Model file for the job. Use its own axes, mm. A direction names the side the tool comes from. Round coordinates to 2 decimals unless told otherwise and drop trailing zeros. Order: outer loops, then holes, each group sorted by start corner. A loop starts at its lowest first (then second) coordinate and runs counter-clockwise, first axis right, second up. Notation, with made-up numbers: (45.25, 65) - (60.25, 65) arc R29 cw to (60.25, 94) - close; hole circle Ø8 at (-26, 0). An arc over 180 degrees is marked (long way). Put each result on its own line as item: value. Start each with the question number.
Item 1: Which spindle directions (+Z, -Z, +X, -X, +Y, -Y) get a long thin tool onto all of the face, cutting with end or side? Do faces 4 (the face through (-73, -25.5, 3)), 5 (the face through (-45, -12, 3)), 6 (the face through (45, -68, 3)), 7 (the face through (-70, 12, 3)), 8 (the face through (15, -68, 3)). Say none if no direction does.
Item 2: Saw through at C-C on y = -33.5. List the corners of the cut face in (x, z).
Item 3: Pin check, flat tips, straight feed: pin 1 Ø2.5 at (y, z) = (12, 3) entering from +X; pin 2 Ø1.5 at (x, z) = (-47, 4) entering from -Y; pin 3 Ø1.5 at (x, z) = (-73.5, 2.5) entering from -Y. Stop position of each tip, or through.
Item 4: Saw through at D-D on x = -49.5. List the corners of the cut face in (y, z), plus the area to 3 significant figures.
Item 5: Saw through at A-A on y = -14. List the corners of the cut face in (x, z), plus the area to 3 significant figures.
Item 6: Mould opens along X. For faces 1 (the face through (72, 4.5, 3)), 2 (the face through (45, -13, 3)), 3 (the face through (-75, -10, 2)) say: pulls with the +X half, pulls with the -X half, needs draft (parallel to the pull), parting line crosses it, or undercut.
Item 7: Saw through at B-B on z = 4.15. List the corners of the cut face in (x, y), plus the area to 4 significant figures.
Item 8: Probe probe 1 along X at (y, z) = (-15, 0.6); probe 2 along X at (y, z) = (11, 3.05); probe 3 along Y at (x, z) = (41, 1). List the from-to ranges inside material, lowest first.
Autodesk Inventor part; units mm, degrees
ref_plane "YZ Plane" through (0, 0, 0) normal (1, 0, 0) x (0, 1, 0)
ref_plane "XZ Plane" through (0, 0, 0) normal (0, 1, 0) x (-1, 0, 0)
ref_plane "XY Plane" through (0, 0, 0) normal (0, 0, 1) x (1, 0, 0)
sketch "Sketch1" plane through (0, 0, 0) normal (0, 0, 1) x (1, 0, 0)
  line L0 (0, 2.8582) -> (0, -2.8582) construction
  line L1 (-5.7775, 0) -> (5.7775, 0) construction
  line L2 (-75, -70.5) -> (75, -70.5)
  line L3 (75, -70.5) -> (75, 70.5)
  line L4 (75, 70.5) -> (-75, 70.5)
  line L5 (-75, 70.5) -> (-75, -70.5)
  line L6 (-75, -70.5) -> (75, 70.5) construction
  line L7 (75, -70.5) -> (-75, 70.5) construction
  point P0 (0, 0)
  point P1 (0, 0)
  dimension "d0" = 150
  dimension "d1" = 141
extrude "Extrusion1" add sketch "Sketch1" along normal blind 5
sketch "Sketch2" plane through (0, 0, 5) normal (0, 0, 1) x (1, 0, 0)
  line L0 (-75, -70.5) -> (75, -70.5)
  line L1 (0, -70.5) -> (-15, -70.5)
  line L2 (-15, -70.5) -> (15, -70.5)
  line L3 (15, -70.5) -> (45, -70.5)
  line L4 (-15, -70.5) -> (-45, -70.5)
  line L5 (-15, -70.5) -> (15, -70.5)
  line L6 (15, -70.5) -> (15, -65.5)
  line L7 (15, -65.5) -> (-15, -65.5)
  line L8 (-15, -65.5) -> (-15, -70.5)
  line L9 (75, -70.5) -> (75, 70.5)
  line L10 (45, -70.5) -> (75, -70.5)
  line L11 (75, -70.5) -> (75, -65.5)
  line L12 (75, -65.5) -> (45, -65.5)
  line L13 (45, -65.5) -> (45, -70.5)
  line L14 (-75, 70.5) -> (-75, -70.5)
  line L15 (-45, -70.5) -> (-75, -70.5)
  line L16 (-75, -70.5) -> (-75, -65.5)
  line L17 (-75, -65.5) -> (-45, -65.5)
  line L18 (-45, -65.5) -> (-45, -70.5)
  line L19 (75, -70.5) -> (75, -55.5)
  line L20 (75, -55.5) -> (75, -25.5)
  line L21 (75, -25.5) -> (75, 4.5)
  line L22 (75, 4.5) -> (75, 34.5)
  line L23 (75, 34.5) -> (75, 64.5)
  line L24 (75, -25.5) -> (70, -25.5)
  line L25 (70, -25.5) -> (70, 4.5)
  line L26 (70, 4.5) -> (75, 4.5)
  line L27 (75, 4.5) -> (75, -25.5)
  line L28 (75, 70.5) -> (-75, 70.5)
  line L29 (75, 34.5) -> (70, 34.5)
  line L30 (70, 34.5) -> (70, 70.5)
  line L31 (70, 70.5) -> (75, 70.5)
  line L32 (75, 70.5) -> (75, 34.5)
  line L33 (-75, -25.5) -> (-70, -25.5)
  line L34 (-70, -25.5) -> (-70, 4.5)
  line L35 (-70, 4.5) -> (-75, 4.5)
  line L36 (-75, 4.5) -> (-75, -25.5)
  line L37 (-75, 34.5) -> (-70, 34.5)
  line L38 (-70, 34.5) -> (-70, 70.5)
  line L39 (-70, 70.5) -> (-75, 70.5)
  line L40 (-75, 70.5) -> (-75, 34.5)
  line L41 (0, 70.5) -> (-15, 70.5)
  line L42 (-15, 70.5) -> (15, 70.5)
  line L43 (15, 70.5) -> (45, 70.5)
  line L44 (-15, 70.5) -> (-45, 70.5)
  line L45 (-75, 70.5) -> (-45, 70.5)
  line L46 (-45, 70.5) -> (-45, 65.5)
  line L47 (-45, 65.5) -> (-75, 65.5)
  line L48 (-75, 65.5) -> (-75, 70.5)
  line L49 (-15, 70.5) -> (15, 70.5)
  line L50 (15, 70.5) -> (15, 65.5)
  line L51 (15, 65.5) -> (-15, 65.5)
  line L52 (-15, 65.5) -> (-15, 70.5)
  line L53 (45, 70.5) -> (75, 70.5)
  line L54 (75, 70.5) -> (75, 65.5)
  line L55 (75, 65.5) -> (45, 65.5)
  line L56 (45, 65.5) -> (45, 70.5)
  line L57 (-75, -25.5) -> (-70, -25.5)
  line L58 (-70, -25.5) -> (-70, -70.5)
  line L59 (-70, -70.5) -> (-75, -70.5)
  line L60 (-75, -70.5) -> (-75, -25.5)
  line L61 (-75, 4.5) -> (-70, 4.5)
  line L62 (-70, 4.5) -> (-70, 34.5)
  line L63 (-70, 34.5) -> (-75, 34.5)
  line L64 (-75, 34.5) -> (-75, 4.5)
  line L65 (70, 34.5) -> (75, 34.5)
  line L66 (75, 34.5) -> (75, 4.5)
  line L67 (75, 4.5) -> (70, 4.5)
  line L68 (70, 4.5) -> (70, 34.5)
  line L69 (70, -25.5) -> (75, -25.5)
  line L70 (75, -25.5) -> (75, -70.5)
  line L71 (75, -70.5) -> (70, -70.5)
  line L72 (70, -70.5) -> (70, -25.5)
  point P0 (0, 0)
  point P1 (75, 4.5)
  point P2 (-70, 70.5)
  point P3 (-75, 4.5)
  point P4 (70, 65.5)
  point P5 (-70, 65.5)
  point P6 (-70, -65.5)
  point P7 (70, -65.5)
  dimension "d4" = 15
  dimension "d5" = 30
  dimension "d6" = 30
  dimension "d7" = 30
  dimension "d8" = 30
  dimension "d9" = 5
  dimension "d10" = 15
  dimension "d11" = 30
  dimension "d14" = 30
  dimension "d15" = 5
  dimension "d16" = 5
  dimension "d17" = 5
  dimension "d24" = 15
  dimension "d25" = 30
  dimension "d26" = 30
  dimension "d27" = 30
  dimension "d28" = 5
  dimension "d32" = 5
  dimension "d33" = 30
  dimension "d34" = 30
extrude "Extrusion2" cut sketch "Sketch2" against normal blind 8 contours L14 L17 L58 L0 | L58 L17 L18 L0 | L14 L33 L58 L17 | L8 L7 L6 L0 | L14 L37 L62 L35 | L14 L28 L38 L47 | L13 L12 L72 L0 | L38 L28 L46 L47 | L72 L12 L9 L0 | L72 L24 L9 L12 | L28 L50 L51 L52 | L68 L29 L9 L26 | L55 L56 L28 L30 | L30 L28 L9 L55
sketch "Sketch3" plane through (0, 0, 5) normal (0, 0, 1) x (1, 0, 0)
  line L0 (-45, -45) -> (45, -45)
  line L1 (45, -45) -> (45, 45)
  line L2 (45, 45) -> (-45, 45)
  line L3 (-45, 45) -> (-45, -45)
  line L4 (-45, -45) -> (45, 45) construction
  line L5 (45, -45) -> (-45, 45) construction
  point P0 (0, 0)
  dimension "d20" = 90
  dimension "d21" = 90
extrude "Extrusion3" cut sketch "Sketch3" against normal blind 8
sketch "Sketch4" plane through (0, 0, 5) normal (0, 0, 1) x (1, 0, 0)
  line L0 (75, 34.5) -> (75, 65.5)
  line L1 (75, 65.5) -> (75, 21.5)
  line L2 (75, 21.5) -> (-125.9097, 21.5)
  line L3 (-125.9097, 21.5) -> (-125.9097, 76.2896)
  line L4 (-125.9097, 76.2896) -> (75, 76.2896)
  line L5 (75, 76.2896) -> (75, 21.5)
  point P0 (0, 0)
  dimension "d29" = 44
extrude "Extrusion4" cut sketch "Sketch4" against normal blind 15
sketch "Sketch5" plane through (45, 21.5, 5) normal (0, 1, 0) x (1, 0, 0)
  line L0 (36.0509, -17.7295) -> (-126.227, -17.7295)
  line L1 (-126.227, -17.7295) -> (-126.227, 31.9582)
  line L2 (-126.227, 31.9582) -> (36.0509, 31.9582)
  line L3 (36.0509, 31.9582) -> (36.0509, -17.7295)
  point P0 (-45, 5)
extrude "Extrusion5" cut sketch "Sketch5" against normal blind 2
properties part number "Plaat achter" material "S235"
Results found:
1. face 4: +Z, -Z, -X, -Y
1. face 5: +Z, -Z, +Y
1. face 6: +Z, -Z, +X, -Y
1. face 7: +Z, -Z, -X, +Y
1. face 8: +Z, -Z, -Y
2. outline: (-70, 0) - (-45, 0) - (-45, 5) - (-70, 5) - close; (45, 0) - (70, 0) - (70, 5) - (45, 5) - close
3. pin 1: stops at x = 70
3. pin 2: stops at y = -65.5
3. pin 3: stops at y = -25.5
4. outline: (-65.5, 0) - (19.5, 0) - (19.5, 5) - (-65.5, 5) - close
4. area: 425 mm²
5. outline: (-75, 0) - (-45, 0) - (-45, 5) - (-75, 5) - close; (45, 0) - (75, 0) - (75, 5) - (45, 5) - close
5. area: 300 mm²
6. face 1: needs draft
6. face 2: undercut
6. face 3: pulls with the -X half
7. outline: (-75, -25.5) - (-70, -25.5) - (-70, -65.5) - (-45, -65.5) - (-45, -70.5) - (-15, -70.5) - (-15, -65.5) - (15, -65.5) - (15, -70.5) - (45, -70.5) - (45, -65.5) - (70, -65.5) - (70, -25.5) - (75, -25.5) - (75, 4.5) - (70, 4.5) - (70, 19.5) - (45, 19.5) - (45, -45) - (-45, -45) - (-45, 19.5) - (-70, 19.5) - (-70, 4.5) - (-75, 4.5) - close
7. area: 6,695 mm²
8. probe 1: x = -75 to -45, 45 to 75
8. probe 2: x = -70 to -45, 45 to 70
8. probe 3: y = -70.5 to -45
